```python
from build123d import *

# Parameters (mm, degrees)
SKETCH6_W           = 96
SKETCH6_H           = 48
BOSS_EXTRUDE1_DEPTH = 6.35
SKETCH2_R           = 48
SKETCH2_R_2         = 1
SKETCH2_R_3         = 19.25
SKETCH2_R_4         = 2.5
BOSS_EXTRUDE2_DEPTH = 6.35
SKETCH2_4_R         = 1
SKETCH2_4_R_2       = 19.25
SKETCH2_4_R_3       = 2.5
CUT_EXTRUDE1_DEPTH  = 6.35
CHAMFER1_SIZE       = 0.5
CHAMFER3_SIZE       = 1
CHAMFER5_SIZE       = 3.4


with BuildPart() as part:
    # Sketch6 → Boss-Extrude1 (new body)
    with BuildSketch(Plane(origin=(0, 0, 0), x_dir=(1, 0, 0), z_dir=(0, 1, 0))):
        with Locations((0, -24)):
            Rectangle(SKETCH6_W, SKETCH6_H)
    extrude(amount=BOSS_EXTRUDE1_DEPTH)

    # Sketch2 → Boss-Extrude2 (add)
    with BuildSketch(Plane(origin=(0, 0, 0), x_dir=(1, 0, 0), z_dir=(0, 1, 0))):
        Circle(SKETCH2_R)
        with Locations((0, -44)):
            Circle(SKETCH2_R_2, mode=Mode.SUBTRACT)
        with Locations((-34.400585229, -27.433551282)):
            Circle(SKETCH2_R_2, mode=Mode.SUBTRACT)
        with Locations(Location((-42.896828136, 9.790921094, 0), (0, 0, 270))):
            Circle(SKETCH2_R_2, mode=Mode.SUBTRACT)
        with Locations(Location((-19.090884521, 39.642630188, 0), (0, 0, 270))):
            Circle(SKETCH2_R_2, mode=Mode.SUBTRACT)
        with Locations(Location((19.090884521, 39.642630188, 0), (0, 0, 270))):
            Circle(SKETCH2_R_2, mode=Mode.SUBTRACT)
        with Locations(Location((42.896828136, 9.790921094, 0), (0, 0, 270))):
            Circle(SKETCH2_R_2, mode=Mode.SUBTRACT)
        with Locations((34.400585229, -27.433551282)):
            Circle(SKETCH2_R_2, mode=Mode.SUBTRACT)
        Circle(SKETCH2_R_3, mode=Mode.SUBTRACT)
        with Locations(Location((23.5, 23.5, 0), (0, 0, 270))):
            Circle(SKETCH2_R_4, mode=Mode.SUBTRACT)
        with Locations((23.5, -23.5)):
            Circle(SKETCH2_R_4, mode=Mode.SUBTRACT)
        with Locations((-23.5, -23.5)):
            Circle(SKETCH2_R_4, mode=Mode.SUBTRACT)
        with Locations(Location((-23.5, 23.5, 0), (0, 0, 270))):
            Circle(SKETCH2_R_4, mode=Mode.SUBTRACT)
    extrude(amount=BOSS_EXTRUDE2_DEPTH)

    # Sketch2_4 → Cut-Extrude1 (cut)
    with BuildSketch(Plane(origin=(0, 0, 0), x_dir=(1, 0, 0), z_dir=(0, 1, 0))):
        with Locations(Location((0, -44, 0), (0, 0, 270))):
            Circle(SKETCH2_4_R)
        with Locations(Location((-34.400585229, -27.433551282, 0), (0, 0, 270))):
            Circle(SKETCH2_4_R)
        with Locations(Location((34.400585229, -27.433551282, 0), (0, 0, 270))):
            Circle(SKETCH2_4_R)
        with Locations(Location((0, 0, 0), (0, 0, 270))):
            Circle(SKETCH2_4_R_2)
        with Locations(Location((23.5, -23.5, 0), (0, 0, 270))):
            Circle(SKETCH2_4_R_3)
        with Locations(Location((-23.5, -23.5, 0), (0, 0, 270))):
            Circle(SKETCH2_4_R_3)
    extrude(amount=CUT_EXTRUDE1_DEPTH, mode=Mode.SUBTRACT)

    # Chamfer1
    chamfer1_edges = [part.edges().sort_by_distance(p)[0] for p in [
        (0, 6.35, 48),
        (48, 6.35, 24),
        (0, 6.35, -48),
        (-48, 6.35, 24),
    ]]
    chamfer(chamfer1_edges, length=CHAMFER1_SIZE)

    # Chamfer3
    chamfer3_edges = [part.edges().sort_by_distance(p)[0] for p in [
        (0, 6.35, -19.25),
    ]]
    chamfer(chamfer3_edges, length=CHAMFER3_SIZE)

    # Chamfer5
    chamfer5_edges = [part.edges().sort_by_distance(p)[0] for p in [
        (-23.5, 0, -26),
        (23.5, 0, -26),
        (-23.5, 0, 21),
        (23.5, 0, 21),
    ]]
    chamfer(chamfer5_edges, length=CHAMFER5_SIZE)


solid = part.part
```
The model under review builds one solid part; all positions refer to its coordinate system, in mm. Round coordinates to 2 decimals unless told otherwise and drop trailing zeros. Write each loop counter-clockwise with the first axis right and the second up, starting at its lowest first coordinate (ties: lowest second). Pieces come first, ordered by that corner, then holes. Notation, with made-up numbers: M -18.75,13 L 14.25,13 A3 ccw 14.25,17 Z; hole C 52,55.5 d9. An arc over 180 degrees is marked long. Use CSV: the item, a comma, the result in double quotes. Start each with the question number.
(1) For line 1 along X through (y, z) = (3.7, 0); line 2 along Z through (x, y) = (3.5, 4.5); line 3 along X through (y, z) = (5.75, -2.5), list the stretches that pass through material, from the lowest coordinate up.
(2) The part is to be moulded in two halves that separate along X. For faces 1 (the face through (25.19, 4.85, -25.34)), 2 (the face through (-48, 3, 24)), 3 (the face through (-1, 0, 21)), 4 (the face through (-18.792, 2.638, -4.173)), say which applies: +X half, -X half, draft (parallel to the pull), parting line (faces both ways), or undercut.
(3) We need section A-A, the plane z = 23.5. State the section outline as (x, y) points.
(4) We need section B-B, the plane y = 1.5. State how many separate pieces and enclosed holes the cut face has, then the cut area to 3 significant figures.
(5) Clearance check with flat-ended pins moving along their axes: P1, Ø8, axis at x = -23.5, z = -23.5, coming from the -Y side; P2, Ø1.8, axis at x = -19.09, z = -39.64, coming from the +Y side; P3, Ø1.5, axis at x = 13, y = 3, coming from the -Z side; P4, Ø6.5, axis at x = 23.5, z = 23.5, coming from the -Y side. State where each tip first meets the part, or that it passes through.
Findings:
1,line 1,"-48 to -19.25, 19.25 to 48"
1,line 2,"-47.87 to -18.93, 18.93 to 48"
1,line 3,"-47.93 to -19.49, 19.49 to 47.93"
2,face 1,"undercut"
2,face 2,"-X half"
2,face 3,"draft"
2,face 4,"undercut"
3,outline,"M -48,0 L -29.4,0 L -26,3.4 L -26,6.35 L -47.5,6.35 L -48,5.85 Z; M -21,3.4 L -17.6,0 L 17.6,0 L 21,3.4 L 21,6.35 L -21,6.35 Z; M 26,3.4 L 29.4,0 L 48,0 L 48,5.85 L 47.5,6.35 L 26,6.35 Z"
4,separate pieces,"1"
4,enclosed holes,"12"
4,area,"6,800 mm^2"
5,P1,"y = 1.9"
5,P2,"through"
5,P3,"z = -46.41"
5,P4,"y = 2.65"
